For this review, use the dimensioned drawing (mm, ordinates from the lowest corner) and the shaded views. Round coordinates to 2 decimals unless told otherwise and drop trailing zeros. Order: outer loops, then holes, each group sorted by start corner. A loop starts at its lowest first (then second) coordinate and runs counter-clockwise, first axis right, second up. Notation, with made-up numbers: (11, 81) -> (45, 81) arc R10 ccw to (45, 96) -> close; hole circle Ø3 at (72.5, -27.5). An arc over 180 degrees is marked (long way). Use a Markdown table: item, result. Add a question column.
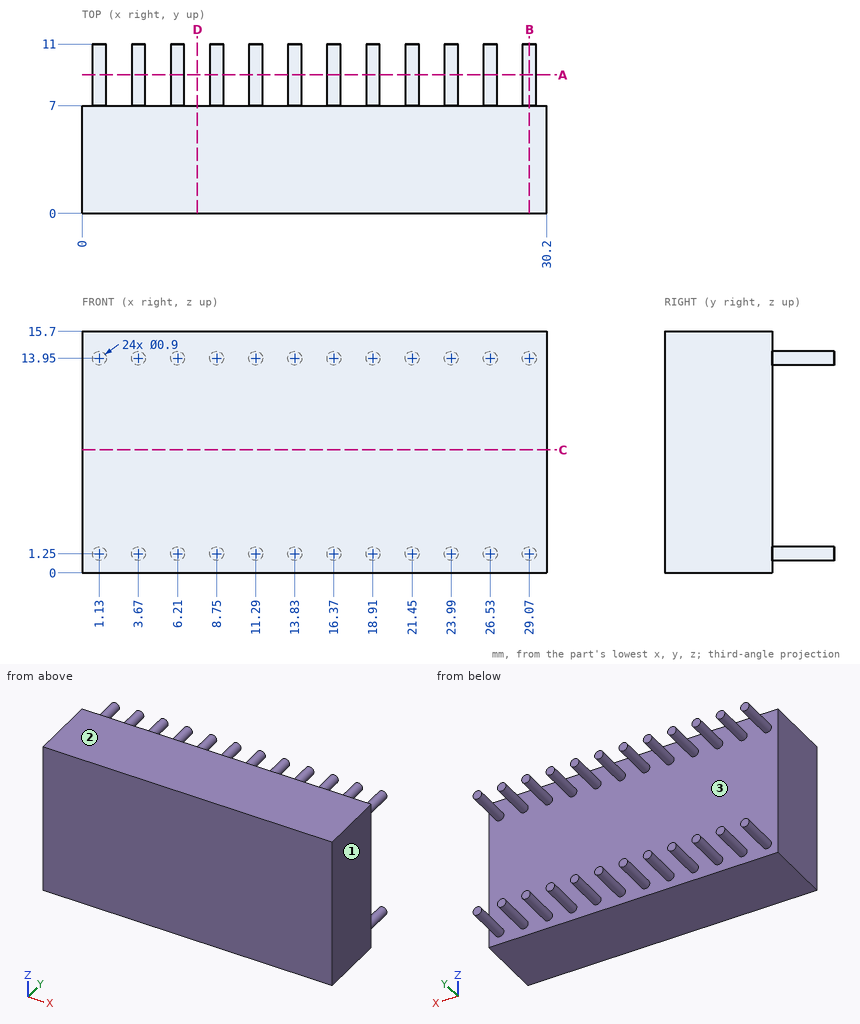
Q1. Add section A-A (y = 9). State how many separate pieces and enclosed holes the cut face has, then the cut area to 3 significant figures.
Q2. Wall thickness on line 1 (Y direction, x = 15, z = 13); line 2 (Z direction, x = 6.5, y = 8.25): over which ranges is each line inside the solid? List them lowest first. Write a range as [from, to].
Q3. Add section B-B (x = 29.07). Write out the cut boundary in (y, z), then the cut area to 3 significant figures.
Q4. Mouldability with a two-part tool opening along Z and no side actions: class the marked faces 1, 2 and 3 as pulls with the +Z half, pulls with the -Z half, needs draft (parallel to the pull), parting line crosses it, or undercut.
Q5. Add section D-D (x = 7.5). Write out the cut boundary in (y, z).
Q6. Add section C-C (z = 8). Write out the cut boundary in (x, y), then the cut area to 3 significant figures.
Report:
| question | item | result |
|---|---|---|
| 1 | separate pieces | 24 |
| 1 | enclosed holes | 0 |
| 1 | area | 15.3 mm² |
| 2 | line 1 | y = [0, 7] |
| 2 | line 2 | z = [0.91, 1.59], [13.61, 14.29] |
| 3 | outline | (0, 0) -> (7, 0) -> (7, 0.8) -> (11, 0.8) -> (11, 1.7) -> (7, 1.7) -> (7, 13.5) -> (11, 13.5) -> (11, 14.4) -> (7, 14.4) -> (7, 15.7) -> (0, 15.7) -> close |
| 3 | area | 117 mm² |
| 4 | face 1 | needs draft |
| 4 | face 2 | pulls with the +Z half |
| 4 | face 3 | undercut |
| 5 | outline | (0, 0) -> (7, 0) -> (7, 15.7) -> (0, 15.7) -> close |
| 6 | outline | (0, 0) -> (30.2, 0) -> (30.2, 7) -> (0, 7) -> close |
| 6 | area | 211 mm² |
